```python
from build123d import *

# Parameters (mm, degrees)
F1_DEPTH = 76.2
F2_R     = 68.4578192755
F3_SIZE  = 5.08
F4_T     = -2.54
F5_R     = 23.8881657529


with BuildPart() as f1:
    # F0 (on Top) → F1 (new body)
    with BuildSketch(Plane.XY):
        Polygon((-147.3665168505, 191.0085547507), (-147.3665168505, -113.7914452493), (24.251197043, -113.7914452493), (18.1496212227, 42.8132099656), (126.6276255479, 42.8132099656), (126.6276255479, 191.0085547507), align=None)
    extrude(amount=F1_DEPTH)

    # F2
    f2_edges = [f1.edges().sort_by_distance(p)[0] for p in [
        (18.149621, 42.81321, 38.1),
    ]]
    fillet(f2_edges, radius=F2_R)

    # F3
    f3_edges = [f1.edges().sort_by_distance(p)[0] for p in [
        (22.585944, -71.050631, 76.2),
    ]]
    chamfer(f3_edges, length=F3_SIZE)

    # F4
    f4_openings = [f1.faces().sort_by_distance(p)[0] for p in [
        (-30.069357, 56.198689, 0),
        (-10.369446, 191.008555, 38.1),
    ]]
    offset(amount=F4_T, openings=f4_openings)

    # F5
    f5_edges = [f1.edges().sort_by_distance(p)[0] for p in [
        (124.087626, 119.976934, 73.66),
    ]]
    fillet(f5_edges, radius=F5_R)


solid = f1.part
```
Verification items for the finished model (mm, model axes). A direction names the side the tool comes from. Give positions to 0.01 mm unless a question says otherwise; leave off trailing zeros. Order: outer loops, then holes, each group sorted by start corner. A loop starts at its lowest first (then second) coordinate and runs counter-clockwise, first axis right, second up. Notation, with made-up numbers: M 67,28.25 L 125,28.25 A15 cw 125,35.25 Z; hole C 55.5,-40 d1. An arc over 180 degrees is marked long. Return JSON: item names as keys, results as strings. Group by question number.
1) Access from +Z, -Z, +X, -X, +Y, -Y to the whole of each face (thin tool, end or side, straight path). Record for faces 4 (the face through (39.5, 21.3, 36.1)), 5 (the face through (39.22, 21.47, 71.44)), 6 (the face through (117.276, 119.2, 66.477)).
2) Go/stop test with flat-tipped pins: pin 1 Ø5 at (y, z) = (22.5, 36.5) entering from +X; pin 2 Ø6 at (x, y) = (45.5, 69) entering from -Z; pin 3 Ø22 at (x, z) = (-95.5, 31) entering from +Y. Record where each tip stops, or that it passes through.
3) Section check D-D on y = -90. Record the cut outline in (x, z).
4) Section check A-A on z = 7. Record the cut outline in (x, y).
5) Mould release check, pull along X, two halves, no side actions. Record for faces 1 (the face through (108, 42.813, 35)), 2 (the face through (22.61, -71.65, 35.06)), 3 (the face through (20.02, -70.41, 34.54)): pulls with the +X half, pulls with the -X half, needs draft (parallel to the pull), parting line crosses it, or undercut.
6) Scan lines: line 1 (X direction, y = -22.5, z = 30.5); line 2 (X direction, y = 74, z = 49.5); line 3 (Y direction, x = 9.5, z = 55.5). Record each from-to range of solid material in increasing order.
7) Section check B-B on y = 93. Record the cut outline in (x, z).
8) Section check C-C on x = -34. Record the cut outline in (y, z), and give its area (3 significant figures).
Answer block:
{
 "1": {"face 4": "+Z, -Z, +X", "face 5": "+Z, +X", "face 6": "-Z, +Y"},
 "2": {"pin 1": "stops at x = 43.27", "pin 2": "stops at z = 73.66", "pin 3": "stops at y = -111.25"},
 "3": {"outline": "M -147.37,0 L -144.83,0 L -144.83,73.66 L 17.19,73.66 L 20.78,70.07 L 20.78,0 L 23.32,0 L 23.32,71.12 L 18.24,76.2 L -147.37,76.2 Z"},
 "4": {"outline": "M -147.37,-113.79 L 24.25,-113.79 L 20.92,-28.31 A68.46 cw 89.33,42.81 L 126.63,42.81 L 126.63,191.01 L 124.09,191.01 L 124.09,45.35 L 89.33,45.35 A71 ccw 18.38,-28.41 L 21.61,-111.25 L -144.83,-111.25 L -144.83,191.01 L -147.37,191.01 Z"},
 "5": {"face 1": "needs draft", "face 2": "pulls with the +X half", "face 3": "undercut"},
 "6": {"line 1": "x = -147.37 to -144.83, 18.4 to 20.94", "line 2": "x = -147.37 to -144.83, 124.09 to 126.63", "line 3": "y = -113.79 to -111.25"},
 "7": {"outline": "M -147.37,0 L -144.83,0 L -144.83,73.66 L 100.2,73.66 A23.89 cw 124.09,49.77 L 124.09,0 L 126.63,0 L 126.63,76.2 L -147.37,76.2 Z"},
 "8": {"outline": "M -113.79,0 L -111.25,0 L -111.25,73.66 L 191.01,73.66 L 191.01,76.2 L -113.79,76.2 Z", "area": "961 mm^2"}
}
